Design review of the part built by this model. Coordinates are the model's own, in mm. A direction names the side the tool comes from. Give positions to 0.01 mm unless a question says otherwise; leave off trailing zeros. Order: outer loops, then holes, each group sorted by start corner. A loop starts at its lowest first (then second) coordinate and runs counter-clockwise, first axis right, second up. Notation, with made-up numbers: (-24.75, 19) - (7.25, 19) arc R17 ccw to (7.25, 35) - close; hole circle Ø1 at (21.25, 18). An arc over 180 degrees is marked (long way). Write each question's results on one line, items separated by ' | '. Start each with the question number.
Autodesk Inventor part; units mm, degrees
ref_plane "YZ Plane" through (0, 0, 0) normal (1, 0, 0) x (0, 1, 0)
ref_plane "XZ Plane" through (0, 0, 0) normal (0, 1, 0) x (-1, 0, 0)
ref_plane "XY Plane" through (0, 0, 0) normal (0, 0, 1) x (1, 0, 0)
sketch "Sketch1" plane through (0, 0, 0) normal (0, 1, 0) x (-1, 0, 0)
  point P0 (0, 0)
sketch "Sketch2" plane through (0, 0, 0) normal (0, 1, 0) x (-1, 0, 0)
  line L0 (0, 0) -> (35, 0)
  line L1 (35, 0) -> (35, -3)
  line L2 (13, -11) -> (35, -3)
  line L3 (13, -11) -> (0, -11)
  line L4 (-3, -9) -> (0, -11)
  line L5 (-3, -9) -> (-11, -9)
  line L6 (-11, -9) -> (-11, -3)
  line L7 (-11, -3) -> (-3, -3)
  line L8 (-3, -3) -> (0, 0)
  dimension "d0" = 35
  dimension "d1" = 3
  dimension "d8" = 6
extrude "Extrusion1" add sketch "Sketch2" along normal blind 20
sketch "Sketch3" plane through (0, 20, 0) normal (0, 1, 0) x (1, 0, 0)
  line L0 (11, 9) -> (11, 3)
  line L1 (11, 6) -> (4, 6)
  circle A0 centre (4, 6) radius 1.5
  dimension "d11" = 7
  dimension "d12" = 3
extrude "Extrusion2" add sketch "Sketch3" along normal blind 3
sketch "Sketch4" plane through (-35, 0, 0) normal (0, 0, 1) x (1, 0, 0)
  line L0 (46, 0) -> (46, 20)
  line L1 (46, 10) -> (28, 10)
  line L2 (28, 10) -> (28, 17.5)
  line L3 (28, 17.5) -> (28, 2.5)
  line L4 (28, 2.5) -> (46, 2.5)
  line L5 (28, 17.5) -> (46, 17.5)
  line L6 (46, 2.5) -> (46, 17.5)
  dimension "d15" = 18
  dimension "d16" = 7.5
  dimension "d17" = 15
extrude "Extrusion3" cut sketch "Sketch4" against normal through all
sketch "Sketch5" plane through (-35, 0, 0) normal (0, 0, 1) x (1, 0, 0)
  line L0 (28, 17.5) -> (35, 17.5)
  line L1 (35, 17.5) -> (35, 20)
  line L2 (0, 20) -> (35, 20)
  line L3 (35, 0) -> (35, 2.5)
  line L4 (35, 2.5) -> (28, 2.5)
  line L5 (28, 2.5) -> (28, 17.5)
  line L6 (0, 0) -> (25, 0)
  line L7 (25, 0.1) -> (25, 19.9)
  line L8 (25, 20) -> (0, 20)
  line L9 (0, 20) -> (0, 0)
  line L10 (34.9, 19.9) -> (34.9, 17.6)
  line L11 (34.9, 17.6) -> (27.9, 17.6)
  line L12 (27.9, 17.6) -> (27.9, 2.4)
  line L13 (27.9, 2.4) -> (34.9, 2.4)
  line L14 (34.9, 2.4) -> (34.9, 0.1)
  line L15 (25, 0.1) -> (0.1, 0.1)
  line L16 (0.1, 0.1) -> (0.1, 19.9)
  line L17 (0.1, 19.9) -> (25, 19.9)
  dimension "d20" = 25
  dimension "d21" = 0.1
extrude "Extrusion4" add sketch "Sketch5" along normal blind 3
properties part number "EE Claw"
Q1. Machinability: for faces 5 (the flat face through (-34.9, 10, 1)), 6 (the flat face through (7, 19, -3)), 7 (the cylindrical face through (5.386, 21.479, -6.575)), 8 (the flat face through (7, 19, -9)), 9 (the flat face through (0, 17.5, -5)), which of the approach directions +Z, -Z, +X, -X, +Y, -Y give a long, thin tool a straight path to every point of the face, cutting with its end or side? Answer none if there is none.
Q2. Add section B-B (z = -6). Give the boundary of the cut face in (x, y), plus the area to 3 significant figures.
Q3. Add section A-A (x = 7.5). Give the boundary of the cut face in (y, z), plus the area to 3 significant figures.
Q4. Draft analysis for pull direction Y (two halves, no side actions). For faces 1 (the flat face through (4, 23, -6)), 2 (the flat face through (-10, 10, 1)), 3 (the flat face through (0, 2.5, -5)), 4 (the flat face through (-22, 0.1, 1)), state which applies: pulls with the +Y half, pulls with the -Y half, needs draft (parallel to the pull), parting line crosses it, or undercut.
Q5. Add section C-C (y = 8). Give the boundary of the cut face in (x, z), plus the area to 3 significant figures.
Q6. For line 1 (Y direction, x = -1, z = -4.5); line 2 (X direction, y = 10, z = 2.75); line 3 (Y direction, x = -8, z = -1.25), list the stretches that pass through material, from the lowest coordinate up. Write a range as [from, to].
Q7. Add section D-D (x = -5.5). Give the boundary of the cut face in (y, z).
Q8. Insertion check: pin 1 Ø1.5 at (y, z) = (5, 1) entering from +X; pin 2 Ø1.5 at (x, y) = (-7, 6.5) entering from +Z; pin 3 Ø5 at (x, z) = (-8.5, -9.5) entering from +Y. Each pin has a flat end and moves straight along its axis. Give the tip position at first contact, or say it passes through.
Verdict:
1) face 5: +Z, -X, +Y, -Y | face 6: +Z, +X, +Y, -Y | face 7: +Y | face 8: -Z, +X, +Y, -Y | face 9: +Z, -Z, +X
2) outline: (-26.75, 0) - (11, 0) - (11, 2.5) - (-7, 2.5) - (-7, 17.5) - (11, 17.5) - (11, 20) - (5.5, 20) - (5.5, 23) - (2.5, 23) - (2.5, 20) - (-26.75, 20) - close | area: 494 mm2
3) outline: (0, -9) - (2.5, -9) - (2.5, -3) - (0, -3) - close; (17.5, -9) - (20, -9) - (20, -3) - (17.5, -3) - close | area: 30.0 mm2
4) face 1: pulls with the +Y half | face 2: needs draft | face 3: undercut | face 4: pulls with the -Y half
5) outline: (-35, -3) - (-13, -11) - (-7, -11) - (-7, 0) - (-10, 0) - (-10, 3) - (-34.9, 3) - (-34.9, 0) - (-35, 0) - close | area: 295 mm2
6) line 1: y = [0, 2.5], [17.5, 20] | line 2: x = [-34.9, -10] | line 3: y = [0, 20]
7) outline: (0, -11) - (2.5, -11) - (2.5, 0) - (0, 0) - close; (17.5, -11) - (20, -11) - (20, 0) - (17.5, 0) - close
8) pin 1: stops at x = -10 | pin 2: stops at z = 0 | pin 3: stops at y = 20
